Print and shaded views of the part. All mm, measured from the part's lowest x, y and z. A direction names the side the tool comes from. Coordinates: 2 decimals unless noted, no trailing zeros. Write each loop counter-clockwise with the first axis right and the second up, starting at its lowest first coordinate (ties: lowest second). Pieces come first, ordered by that corner, then holes. Notation, with made-up numbers: (69.5, 64.25) -> (90.5, 64.25) arc R22 ccw to (90.5, 89.25) -> close; hole circle Ø6 at (70, -15). An arc over 180 degrees is marked (long way). Write item = value, one per line.
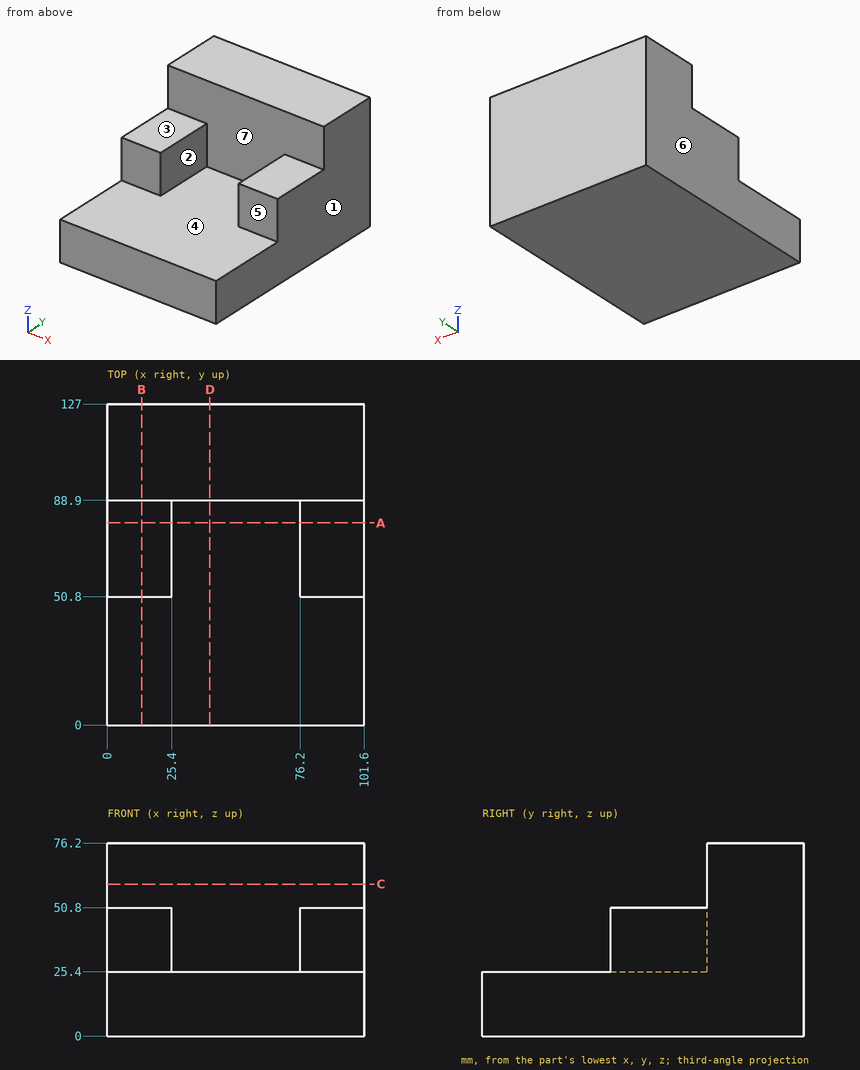
Q1. Which spindle directions (+Z, -Z, +X, -X, +Y, -Y) get a long thin tool onto all of the face, cutting with end or side? Do the marked faces 1, 2 and 3. Say none if no direction does.
Model answer:
face_1 = +Z, -Z, +X, +Y, -Y
face_2 = +Z, -Y
face_3 = +Z, +X, -X, -Y
Q2. Saw through at D-D on x = 40.5. Give the cut face in (y, z).
Model answer:
outline = (0, 0) -> (127, 0) -> (127, 76.2) -> (88.9, 76.2) -> (88.9, 25.4) -> (0, 25.4) -> close
Q3. Saw through at C-C on z = 60. Give the cut face in (x, y).
Model answer:
outline = (0, 88.9) -> (101.6, 88.9) -> (101.6, 127) -> (0, 127) -> close
Q4. Mould opens along X. For the marked faces 4, 5, 6 and 7 say: released by +X, released by -X, zero draft, split by the parting line, or undercut.
Model answer:
face_4 = undercut
face_5 = zero draft
face_6 = released by -X
face_7 = undercut
Q5. Saw through at A-A on y = 80. Give the cut face in (x, z), and give its area (3 significant figures).
Model answer:
outline = (0, 0) -> (101.6, 0) -> (101.6, 50.8) -> (76.2, 50.8) -> (76.2, 25.4) -> (25.4, 25.4) -> (25.4, 50.8) -> (0, 50.8) -> close
area = 3,870 mm²
Q6. Pin check, flat tips, straight feed: pin 1 (7.5 mm diameter, centred on x = 91, z = 32.5, fed in from -Y); pin 2 (12.5 mm diameter, centred on x = 90.5, y = 74.5, fed in from +Z); pin 3 (2 mm diameter, centred on x = 91.5, y = 26.5, fed in from +Z); pin 4 (8 mm diameter, centred on x = 24.5, y = 104, fed in from -Z). Stop position of each tip, or through.
Model answer:
pin_1 = 50.8
pin_2 = 50.8
pin_3 = 25.4
pin_4 = 0
Q7. Saw through at B-B on x = 13.5. Give the cut face in (y, z), and give its area (3 significant figures).
Model answer:
outline = (0, 0) -> (127, 0) -> (127, 76.2) -> (88.9, 76.2) -> (88.9, 50.8) -> (50.8, 50.8) -> (50.8, 25.4) -> (0, 25.4) -> close
area = 6,130 mm²
Q8. Probe line 1 (Z direction, x = 73.5, y = 33); line 2 (Y direction, x = 83.5, z = 38); line 3 (Y direction, x = 33.5, z = 39). List the from-to ranges inside material, lowest first. Write a range as from..to.
Model answer:
line_1 = 0..25.4
line_2 = 50.8..127
line_3 = 88.9..127
